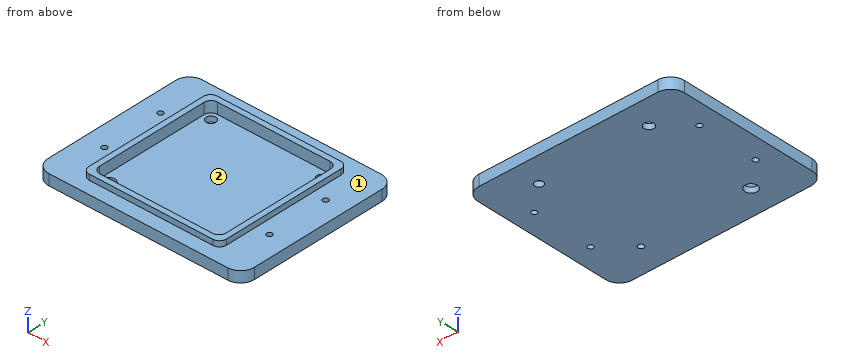
Autodesk Fusion 360 part; units mm, degrees
sketch "스케치1" plane through (0, 0, 0) normal (0, 0, 1) x (1, 0, 0)
  line L0 (-63.1023, 51.7762) -> (86.8977, 51.7762)
  line L1 (86.8977, 51.7762) -> (86.8977, -68.2238)
  line L2 (86.8977, -68.2238) -> (-63.1023, -68.2238)
  line L3 (-63.1023, -68.2238) -> (-63.1023, 51.7762)
  line L4 (-63.1023, -8.2238) -> (86.8977, -8.2238) construction
  point P0 (-63.1023, -8.2238)
  point P1 (86.8977, -8.2238)
  point P2 (11.8977, -8.2238)
  dimension "d1" = 150
  dimension "d2" = 120
sketch "스케치3" plane through (0, 0, 0) normal (0, 0, 1) x (1, 0, 0)
extrude "돌출2" add sketch "스케치1" along normal blind 8
sketch "스케치4" plane through (0, 0, 8) normal (0, 0, 1) x (-1, 0, 0)
  line L0 (63.1023, 68.2238) -> (-86.8977, 68.2238)
  line L1 (-86.8977, 68.2238) -> (-86.8977, -51.7762)
  line L2 (-86.8977, -51.7762) -> (63.1023, -51.7762)
  line L3 (63.1023, -51.7762) -> (63.1023, 68.2238)
  line L4 (38.1023, -41.7762) -> (-61.8977, -41.7762)
  line L5 (-61.8977, -41.7762) -> (-61.8977, 58.2238)
  line L6 (-61.8977, 58.2238) -> (38.1023, 58.2238)
  line L7 (38.1023, 58.2238) -> (38.1023, -41.7762)
  line L8 (34.1023, -37.7762) -> (-57.8977, -37.7762)
  line L9 (-57.8977, -37.7762) -> (-57.8977, 54.2238)
  line L10 (-57.8977, 54.2238) -> (34.1023, 54.2238)
  line L11 (34.1023, 54.2238) -> (34.1023, -37.7762)
  line L12 (63.1023, -51.7762) -> (-86.8977, -51.7762)
  line L13 (-86.8977, 68.2238) -> (63.1023, 68.2238)
  line L14 (-11.8977, -51.7762) -> (-11.8977, 68.2238) construction
  line L15 (63.1023, 68.2238) -> (63.1023, -51.7762) construction
  line L16 (63.1023, 8.2238) -> (-86.8977, 8.2238) construction
  line L17 (-11.8977, -41.7762) -> (-11.8977, 58.2238) construction
  line L18 (38.1023, 8.2238) -> (-61.8977, 8.2238) construction
  line L19 (34.1023, 8.2238) -> (-57.8977, 8.2238) construction
  point P0 (-11.8977, -51.7762)
  point P1 (-11.8977, 68.2238)
  point P2 (63.1023, 8.2238)
  point P3 (-86.8977, 8.2238)
  point P4 (-11.8977, -41.7762)
  point P5 (-11.8977, 58.2238)
  point P6 (38.1023, 8.2238)
  point P7 (-61.8977, 8.2238)
  point P8 (-11.8977, 8.2238)
  point P9 (34.1023, 8.2238)
  point P10 (-57.8977, 8.2238)
  point P11 (-11.8977, 8.2238)
  point P12 (-11.8977, 8.2238)
  dimension "d9" = 100
  dimension "d10" = 100
  dimension "d11" = 92
  dimension "d12" = 92
extrude "돌출3" add sketch "스케치4" along normal blind 4 contours L4 L5 L6 L7
extrude "돌출4" cut 1 faces at (-3.4356, 7.1096, 8) along direction (0, 0, -1) blind 4
sketch "스케치6" plane through (0, 0, 0) normal (0, 0, 1) x (1, 0, 0)
sketch "스케치7" plane through (0, 0, 0) normal (0, 0, 1) x (1, 0, 0)
  line L0 (71.8977, 13.7762) -> (-48.1023, 13.7762) construction
  line L1 (-48.1023, 13.7762) -> (-48.1023, -30.2238) construction
  line L2 (-48.1023, -30.2238) -> (71.8977, -30.2238) construction
  line L3 (71.8977, -30.2238) -> (71.8977, 13.7762) construction
  line L4 (71.8977, -8.2238) -> (-48.1023, -8.2238) construction
  circle A0 centre (71.8977, 13.7762) radius 2
  circle A1 centre (71.8977, -30.2238) radius 2
  circle A2 centre (-48.1023, 13.7762) radius 2
  circle A3 centre (-48.1023, -30.2238) radius 2
  point P0 (71.8977, -8.2238)
  point P1 (-48.1023, -8.2238)
  point P2 (11.8977, -8.2238)
  point P3 (11.8977, -8.2238)
  dimension "d17" = 120
  dimension "d18" = 44
  dimension "d19" = 4
  dimension "d20" = 4
extrude "돌출5" cut sketch "스케치7" along normal blind 10
sketch "스케치8" plane through (0, 0, 4) normal (0, 0, 1) x (-1, 0, 0)
  line L0 (-57.8977, 54.2238) -> (-57.8977, -37.7762)
  line L1 (-57.8977, -37.7762) -> (34.1023, -37.7762)
  line L2 (34.1023, -37.7762) -> (34.1023, 54.2238)
  line L3 (34.1023, 54.2238) -> (-57.8977, 54.2238)
  line L4 (28.1023, -31.7762) -> (-51.8977, -31.7762) construction
  line L5 (-51.8977, -31.7762) -> (-51.8977, 48.2238) construction
  line L6 (-51.8977, 48.2238) -> (28.1023, 48.2238) construction
  line L7 (28.1023, 48.2238) -> (28.1023, -31.7762) construction
  line L8 (34.1023, 8.2238) -> (-57.8977, 8.2238) construction
  line L9 (28.1023, 8.2238) -> (-51.8977, 8.2238) construction
  circle A0 centre (28.1023, -31.7762) radius 3.5748
  circle A1 centre (-51.8977, -31.7762) radius 3.0869
  circle A2 centre (-51.8977, 48.2238) radius 2.1374
  circle A3 centre (28.1023, 48.2238) radius 4.474
  point P0 (34.1023, 8.2238)
  point P1 (-57.8977, 8.2238)
  point P2 (-11.8977, 8.2238)
  point P3 (28.1023, 8.2238)
  point P4 (-51.8977, 8.2238)
  point P5 (-11.8977, 8.2238)
  dimension "d23" = 80
  dimension "d24" = 80
extrude "돌출6" cut sketch "스케치8" against normal blind 5 contours A0 | A1 | A2 | A3
fillet "모깎기6" radius 10 1 edges at (86.8977, -68.2238, 4)
fillet "모깎기7" radius 10 1 edges at (86.8977, 51.7762, 4)
fillet "모깎기8" radius 5 1 edges at (61.8977, -58.2238, 10)
fillet "모깎기9" radius 5 1 edges at (61.8977, 41.7762, 10)
fillet "모깎기10" radius 5 1 edges at (-38.1023, -58.2238, 10)
fillet "모깎기11" radius 5 1 edges at (-38.1023, 41.7762, 10)
fillet "모깎기12" radius 10 1 edges at (-63.1023, -68.2238, 4)
fillet "모깎기13" radius 10 1 edges at (-63.1023, 51.7762, 4)
fillet "모깎기14" radius 5 1 edges at (57.8977, -54.2238, 8)
fillet "모깎기15" radius 5 1 edges at (57.8977, 37.7762, 8)
fillet "모깎기16" radius 5 1 edges at (-34.1023, 37.7762, 8)
fillet "모깎기17" radius 5 1 edges at (-34.1023, -54.2238, 8)
thread "스레드1"
thread "스레드2"
thread "스레드3"
thread "스레드4"
thread "스레드5"
thread "스레드6"
thread "스레드7"
thread "스레드8"
fillet "모깎기1" [suppressed]
fillet "모깎기2" [suppressed]
fillet "모깎기3" [suppressed]
fillet "모깎기4" [suppressed]
fillet "모깎기5" [suppressed]
sketch "스케치5" plane through (0, 0, 8) normal (0, 0, 1) x (-1, 0, 0)
  line L0 (63.1023, 68.2238) -> (-86.8977, 68.2238)
  line L1 (-86.8977, 68.2238) -> (-86.8977, -51.7762)
  line L2 (-86.8977, -51.7762) -> (63.1023, -51.7762)
  line L3 (63.1023, -51.7762) -> (63.1023, 68.2238)
  line L4 (38.1023, 58.2238) -> (38.1023, -41.7762)
  line L5 (38.1023, -41.7762) -> (-61.8977, -41.7762)
  line L6 (-61.8977, -41.7762) -> (-61.8977, 58.2238)
  line L7 (-61.8977, 58.2238) -> (38.1023, 58.2238)
  line L8 (52.6316, -44.9948) -> (-78.4313, -44.9948) construction
  line L9 (-78.4313, -44.9948) -> (-78.4313, 47.678) construction
  line L10 (-78.4313, 47.678) -> (52.6316, 47.678) construction
  line L11 (52.6316, 47.678) -> (52.6316, -44.9948) construction
extrude "돌출1" [suppressed]
sketch "스케치2" plane through (0, 0, 8) normal (0, 0, 1) x (-1, 0, 0)
  line L0 (63.1023, 48.2238) -> (-86.8977, 48.2238)
  line L1 (-86.8977, 48.2238) -> (-86.8977, -51.7762)
  line L2 (-86.8977, -51.7762) -> (63.1023, -51.7762)
  line L3 (63.1023, -51.7762) -> (63.1023, 48.2238)
  line L4 (40.9967, -38.1097) -> (-57.0033, -38.1097)
  line L5 (-57.0033, -38.1097) -> (-57.0033, 32.143)
  line L6 (-57.0033, 32.143) -> (40.9967, 32.143)
  line L7 (40.9967, 32.143) -> (40.9967, -38.1097)
  line L8 (26.9462, -28.1011) -> (-55, -28.1011)
  line L9 (-55, -28.1011) -> (-55, 20)
  line L10 (-55, 20) -> (26.9462, 20)
  line L11 (26.9462, 20) -> (26.9462, -28.1011)
  dimension "d5" = 98
  dimension "d6" = 70.2526
Read the model definition and answer for the solid it produces. Units are mm, in the model's axes. Face numbers are marked on the shaded views. Coordinates: 2 decimals unless noted, no trailing zeros. Loops run counter-clockwise (first coordinate to the right, second up) from the corner with the lowest first, then second, coordinate; pieces in that order, holes last. Notation, with made-up numbers: (9, 44.25) - (34, 44.25) arc R16 cw to (34, 73.25) - close; hole circle Ø5 at (-30, -22). An arc over 180 degrees is marked (long way). Answer in a Markdown table with one row per item.
1. Find section A-A, the plane x = -0.5. Write down the section's boundary in (y, z).
Conclusion:
| item | result |
|---|---|
| outline | (-68.22, 0) - (51.78, 0) - (51.78, 8) - (41.78, 8) - (41.78, 12) - (37.78, 12) - (37.78, 4) - (-54.22, 4) - (-54.22, 12) - (-58.22, 12) - (-58.22, 8) - (-68.22, 8) - close |
2. Given pin 1 (3 mm diameter, centred on x = -45.5, y = -47.5, fed in from +Z); pin 2 (1.5 mm diameter, centred on x = 41.5, z = 9, fed in from -Y); pin 3 (11.5 mm diameter, centred on x = -28.1, y = 31.78, fed in from +Z), each flat-ended and moving along its own axis, determine where each tip first touches the part or whether it passes through.
Conclusion:
| item | result |
|---|---|
| pin 1 | stops at z = 8 |
| pin 2 | stops at y = -58.22 |
| pin 3 | stops at z = 4 |
3. Determine the mould class of the marked faces 1 and 2 for opening direction Y: +Y half, -Y half, draft (parallel to the pull), parting line (faces both ways), or undercut.
Conclusion:
| item | result |
|---|---|
| face 1 | draft |
| face 2 | undercut |
4. Find section C-C, the plane y = 44.5. Write down the section's boundary in (x, z), then the cut area to 3 significant figures.
Conclusion:
| item | result |
|---|---|
| outline | (-62.72, 0) - (86.52, 0) - (86.52, 8) - (-62.72, 8) - close |
| area | 1,190 mm² |
5. Straight lines are drawn through the part: line 1 (X direction, y = -13, z = 8.25); line 2 (Y direction, x = -24.5, z = 6.5); line 3 (Y direction, x = -9.5, z = 11). For each, find the intervals that lie inside material, in ascending order.
Conclusion:
| item | result |
|---|---|
| line 1 | x = -38.1 to -34.1, 57.9 to 61.9 |
| line 2 | y = -68.22 to -54.22, 37.78 to 51.78 |
| line 3 | y = -58.22 to -54.22, 37.78 to 41.78 |
6. Find section B-B, the plane z = 10.25. Write down the section's boundary in (x, y).
Conclusion:
| item | result |
|---|---|
| outline | (-38.1, -53.22) arc R5 ccw to (-33.1, -58.22) - (56.9, -58.22) arc R5 ccw to (61.9, -53.22) - (61.9, 36.78) arc R5 ccw to (56.9, 41.78) - (-33.1, 41.78) arc R5 ccw to (-38.1, 36.78) - close; hole (-34.1, -49.22) arc R5 ccw to (-29.1, -54.22) - (52.9, -54.22) arc R5 ccw to (57.9, -49.22) - (57.9, 32.78) arc R5 ccw to (52.9, 37.78) - (-29.1, 37.78) arc R5 ccw to (-34.1, 32.78) - close |
